Could you check a few things on this drawing? It's one solid part, dimensions in mm from its lowest x, y, z. A direction names the side the tool comes from. Give positions to 0.01 mm unless a question says otherwise; leave off trailing zeros. Order: outer loops, then holes, each group sorted by start corner. A loop starts at its lowest first (then second) coordinate and runs counter-clockwise, first axis right, second up. Notation, with made-up numbers: M 56.5,2 L 60.5,2 A24 cw 60.5,26 Z; hole C -24.5,44.25 d7. An arc over 180 degrees is marked long. Use one line per item in the form item = value.
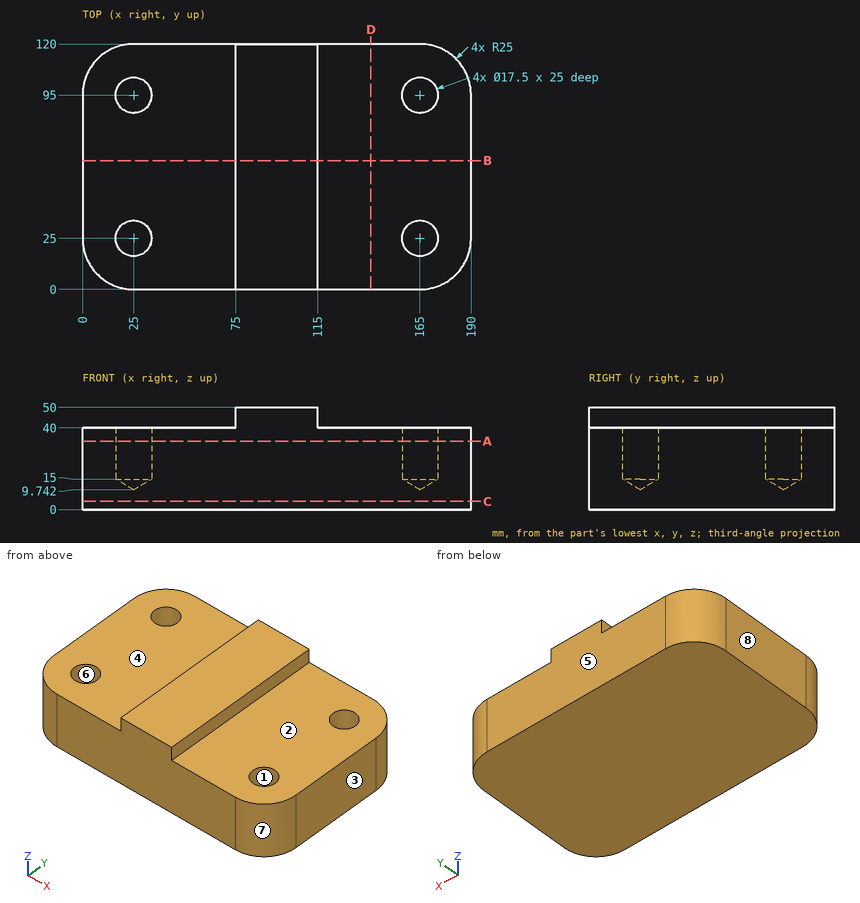
Q1. Thinking about a two-plate mould opening in Y: for the marked faces 6, 7 and 8, which applies, +Y half, -Y half, draft (parallel to the pull), parting line (faces both ways), or undercut?
Found:
face_6 = undercut
face_7 = -Y half
face_8 = draft
Q2. I want a section at A-A on z = 33.5. Write out the boundary of the cut face in (x, y).
Found:
outline = M 0,25 A25 ccw 25,0 L 165,0 A25 ccw 190,25 L 190,95 A25 ccw 165,120 L 25,120 A25 ccw 0,95 Z; hole C 25,25 d17.5; hole C 25,95 d17.5; hole C 165,25 d17.5; hole C 165,95 d17.5
Q3. I want a section at B-B on y = 63. Write out the boundary of the cut face in (x, z), then the cut area to 3 significant figures.
Found:
outline = M 0,0 L 190,0 L 190,40 L 115,40 L 115,50 L 75,50 L 75,40 L 0,40 Z
area = 8,000 mm²
Q4. I need wall thicknesses on L1, parallel to Y at x = 25, z = 33; L2, parallel to Y at x = 23.5, z = 30.5 (1 decimal); L3, parallel to X at y = 103, z = 24.5 (1 decimal). Which ranges of each line are inside material? Lowest first, please.
Found:
L1 = 0 to 16.25, 33.75 to 86.25, 103.75 to 120
L2 = 0 to 16.4, 33.6 to 86.4, 103.6 to 120
L3 = 1.3 to 21.5, 28.5 to 161.5, 168.5 to 188.7
Q5. I want a section at C-C on z = 4. Write out the boundary of the cut face in (x, y), then the cut area to 3 significant figures.
Found:
outline = M 0,25 A25 ccw 25,0 L 165,0 A25 ccw 190,25 L 190,95 A25 ccw 165,120 L 25,120 A25 ccw 0,95 Z
area = 22,300 mm²
Q6. I want a section at D-D on x = 141. Write out the boundary of the cut face in (y, z), then the cut area to 3 significant figures.
Found:
outline = M 0,0 L 120,0 L 120,40 L 0,40 Z
area = 4,800 mm²
Q7. I'm going to push flat-ended pins straight in: pin 1 Ø16 at (x, y) = (25, 95) entering from +Z; pin 2 Ø5 at (y, z) = (84.5, 45) entering from +X; pin 3 Ø22.5 at (x, y) = (144.5, 57.5) entering from +Z. Where does each tip first touch, or does it pass through?
Found:
pin_1 = 14.55
pin_2 = 115
pin_3 = 40
Q8. On a 3-axis mill with a long thin cutter (end or side, diameter ignored), from which of +Z, -Z, +X, -X, +Y, -Y can I reach the whole of each face in a straight line? I mean the marked faces 1, 2, 3, 4 and 5. Say none if no direction works.
Found:
face_1 = +Z
face_2 = +Z, +X, +Y, -Y
face_3 = +Z, -Z, +X, +Y, -Y
face_4 = +Z, -X, +Y, -Y
face_5 = +Z, -Z, +X, -X, +Y
